Autodesk Inventor part; units mm, degrees
ref_plane "YZ Plane" through (0, 0, 0) normal (1, 0, 0) x (0, 1, 0)
ref_plane "XZ Plane" through (0, 0, 0) normal (0, 1, 0) x (-1, 0, 0)
ref_plane "XY Plane" through (0, 0, 0) normal (0, 0, 1) x (1, 0, 0)
sketch "Sketch1" plane through (0, 0, 0) normal (0, 1, 0) x (-1, 0, 0)
  line L0 (0, 0) -> (42.3, 0) construction
  line L1 (42.3, 0) -> (42.3, -42.3) construction
  line L2 (42.3, -42.3) -> (0, -42.3) construction
  line L3 (0, -42.3) -> (0, 0) construction
  circle A0 centre (36.65, -5.65) radius 1.7
  circle A1 centre (36.65, -36.65) radius 1.7
  circle A2 centre (5.65, -5.65) radius 1.7
  circle A3 centre (5.65, -36.65) radius 1.7
  line L4 (5.65, -5.65) -> (5.65, -36.65) construction
  line L5 (5.65, -36.65) -> (36.65, -36.65) construction
  line L6 (36.65, -36.65) -> (36.65, -5.65) construction
  line L7 (36.65, -5.65) -> (5.65, -5.65) construction
  circle A4 centre (36.65, -5.65) radius 3
  circle A5 centre (36.65, -36.65) radius 3
  circle A6 centre (5.65, -36.65) radius 3
  circle A7 centre (5.65, -5.65) radius 3
  dimension "d0" = 42.3
  dimension "d1" = 42.3
  dimension "d2" = 3.4
  dimension "d3" = 3.4
  dimension "d4" = 31
  dimension "d5" = 3.4
  dimension "d6" = 3.4
  dimension "d8" = 31
  dimension "d9" = 5.65
  dimension "d10" = 5.65
  dimension "d11" = 31
  dimension "d12" = 6
  dimension "d13" = 6
  dimension "d14" = 6
  dimension "d15" = 6
extrude "Extrusion1" add sketch "Sketch1" along normal blind 4
sketch "Sketch2" plane through (-36.65, 4, -5.65) normal (0, 1, 0) x (1, 0, 0)
  line L0 (-5.65, -5.65) -> (-5.65, 36.65) construction
  line L1 (36.65, -5.65) -> (-5.65, -5.65) construction
  line L2 (-5.65, 36.65) -> (36.65, 36.65) construction
  line L3 (36.65, 36.65) -> (36.65, -5.65) construction
  line L4 (-5.65, -5.65) -> (36.65, 36.65) construction
  line L5 (-5.65, 36.65) -> (36.65, -5.65) construction
  line L6 (24.5, 4.5) -> (6.5, 4.5)
  line L7 (6.5, 4.5) -> (6.5, 26.5)
  line L8 (6.5, 26.5) -> (24.5, 26.5)
  line L9 (24.5, 26.5) -> (24.5, 4.5)
  line L10 (24.5, 4.5) -> (6.5, 26.5) construction
  line L11 (6.5, 4.5) -> (24.5, 26.5) construction
  circle A0 centre (10, 6.5) radius 1.4
  circle A1 centre (10, 24.5) radius 1.4
  circle A2 centre (21, 24.5) radius 1.4
  circle A3 centre (21, 6.5) radius 1.4
  line L12 (10, 24.5) -> (21, 24.5) construction
  line L13 (21, 24.5) -> (21, 6.5) construction
  line L14 (21, 6.5) -> (10, 6.5) construction
  line L15 (10, 6.5) -> (10, 24.5) construction
  line L16 (21, 6.5) -> (21, 4.5) construction
  line L17 (21, 24.5) -> (21, 26.5) construction
  line L18 (10, 6.5) -> (6.5, 6.5) construction
  line L19 (21, 6.5) -> (24.5, 6.5) construction
  circle A4 centre (0, 0) radius 3
  circle A5 centre (0, 31) radius 3
  circle A6 centre (31, 31) radius 3
  circle A7 centre (31, 0) radius 3
  line L20 (11.7705, 4.5) -> (1.7076, -2.4666)
  circle A8 centre (0, 0) radius 3 construction
  line L21 (6.5, 8.1488) -> (-1.7076, 2.4666)
  circle A9 centre (0, 31) radius 3
  line L22 (-1.7076, 28.5334) -> (6.5, 22.8512)
  line L23 (11.7705, 26.5) -> (1.7076, 33.4666)
  line L24 (6.5, 26.5) -> (0, 31) construction
  line L25 (6.5, 4.5) -> (0, 0) construction
  line L26 (24.5, 4.5) -> (31, 0) construction
  line L27 (19.2295, 4.5) -> (29.2924, -2.4666)
  circle A10 centre (31, 0) radius 3
  line L28 (32.7076, 2.4666) -> (24.5, 8.1488)
  line L29 (24.5, 26.5) -> (31, 31) construction
  line L30 (19.2295, 26.5) -> (29.2924, 33.4666)
  line L31 (24.5, 22.8512) -> (32.7076, 28.5334)
  circle A11 centre (31, 31) radius 3
  arc A12 (1.7076, 33.4666) -> (-1.7076, 28.5334) centre (0, 31) ccw
  arc A13 (32.7076, 28.5334) -> (29.2924, 33.4666) centre (31, 31) ccw
  arc A14 (29.2924, -2.4666) -> (32.7076, 2.4666) centre (31, 0) ccw
  arc A15 (-1.7076, 2.4666) -> (1.7076, -2.4666) centre (0, 0) ccw
  circle A16 centre (0, 0) radius 1.7
  circle A17 centre (0, 31) radius 1.7
  circle A18 centre (31, 31) radius 1.7
  circle A19 centre (31, 0) radius 1.7
  circle A20 centre (31, 0) radius 1.7
  circle A21 centre (31, 31) radius 1.7
  circle A22 centre (0, 0) radius 1.7
  circle A23 centre (0, 31) radius 1.7
  point P0 (15.5, 15.5)
  dimension "d18" = 18
  dimension "d19" = 22
  dimension "d20" = 2.8
  dimension "d21" = 2.8
  dimension "d22" = 2.8
  dimension "d23" = 2.8
  dimension "d24" = 11
  dimension "d25" = 18
extrude "Extrusion2" add sketch "Sketch2" along normal blind 3
properties part number "AdapterBoardNema17Mount"
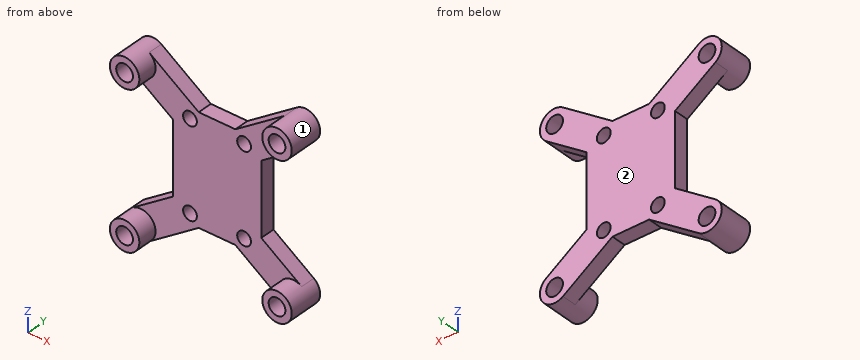
For this review, take the finished solid that the model builds, in its own axes (mm). Face numbers are marked on the shaded views. Round coordinates to 2 decimals unless told otherwise and drop trailing zeros. Write each loop counter-clockwise with the first axis right and the second up, starting at its lowest first coordinate (ties: lowest second). Pieces come first, ordered by that corner, then holes.
1) Mouldability with a two-part tool opening along X and no side actions: class the marked faces 1 and 2 as +X half, -X half, draft (parallel to the pull), parting line (faces both ways), or undercut.
Answer below:
face 1: undercut
face 2: draft
2) Insertion check: pin 1 Ø3 at (x, z) = (-36.65, -36.65) entering from +Y; pin 2 Ø10.5 at (x, z) = (-13.5, -17.5) entering from -Y; pin 3 Ø1 at (y, z) = (6, -13.5) entering from -X; pin 4 Ø4 at (y, z) = (5, -32) entering from -X. Each pin has a flat end and moves straight along its axis. Give the tip position at first contact, or say it passes through.
Answer below:
pin 1: passes through
pin 2: stops at y = 4
pin 3: stops at x = -31.3
pin 4: stops at x = -38.09
3) Take a section at B-B on y = 2.5. Give the boundary of the cut face in (x, z).
Answer below:
outline: circle Ø6 at (-36.65, -36.65); circle Ø6 at (-36.65, -5.65); circle Ø6 at (-5.65, -36.65); circle Ø6 at (-5.65, -5.65); hole circle Ø3.4 at (-36.65, -36.65); hole circle Ø3.4 at (-36.65, -5.65); hole circle Ø3.4 at (-5.65, -36.65); hole circle Ø3.4 at (-5.65, -5.65)
4) Take a section at D-D on z = -12.15. Give the boundary of the cut face in (x, y), then the cut area to 3 significant figures.
Answer below:
outline: (-32.53, 4) - (-28.05, 4) - (-28.05, 7) - (-32.53, 7) - close; (-25.25, 4) - (-17.05, 4) - (-17.05, 7) - (-25.25, 7) - close; (-14.25, 4) - (-9.77, 4) - (-9.77, 7) - (-14.25, 7) - close
area: 51.5 mm2
5) Take a section at A-A on y = 6. State how many separate pieces and enclosed holes the cut face has, then the cut area to 3 significant figures.
Answer below:
separate pieces: 1
enclosed holes: 8
area: 620 mm2
6) For line 1 along Z through (x, y) = (-5.65, 2.6); line 2 along X through (y, z) = (4.7, -12.15), list the stretches that pass through material, from the lowest coordinate up.
Answer below:
line 1: z = -39.65 to -38.35, -34.95 to -33.65, -8.65 to -7.35, -3.95 to -2.65
line 2: x = -32.53 to -28.05, -25.25 to -17.05, -14.25 to -9.77
